from build123d import *

# Parameters (mm, degrees)
BASPROSKE_W         = 4.7625
BASPROSKE_H         = 14
TOOTHCUT_DEPTH      = 21.36372771
TEETHCUTS_COUNT     = 12
TEETHCUTS_ANGLE     = 330
BORSKE_R            = 2.6035
BORE_DEPTH          = 50.0000508
BOSS_EXTRUDE1_DEPTH = 13.99999994
SKETCH2_R           = 2.6035
CUT_EXTRUDE1_DEPTH  = 27.882327142
SKETCH3_R           = 2.5019
CUT_EXTRUDE2_DEPTH  = 32.693338104


with BuildPart() as part:
    # BasProSke → Base-Revolve (revolve)
    with BuildSketch(Plane(origin=(0, 0, 0), x_dir=(1, 0, 0), z_dir=(0, 1, 0)), mode=Mode.PRIVATE) as base_revolve_sk:
        with Locations((2.38125, 7)):
            Rectangle(BASPROSKE_W, BASPROSKE_H)
    revolve(base_revolve_sk.sketch.rotate(Axis((-10, 0, 0), (1, 0, 0)), 180), axis=Axis((-10, 0, 0), (1, 0, 0)))

    # TooCutSke → ToothCut (cut, through all)
    with BuildSketch(Plane(origin=(0, 0, 0), x_dir=(0, 0, -1), z_dir=(1, 0, 0))):
        with BuildLine():
            ThreePointArc((1.111908866, 9.433698091), (0, 9.499), (-1.111908866, 9.433698091))
            ThreePointArc((-1.111908866, 9.433698091), (-1.651516138, 11.821129337), (-3.298149691, 13.632096456))
            ThreePointArc((-3.298149691, 13.632096456), (0, 14.0254), (3.298149691, 13.632096456))
            ThreePointArc((3.298149691, 13.632096456), (1.651516138, 11.821129337), (1.111908866, 9.433698091))
        make_face()
    toothcut = extrude(amount=TOOTHCUT_DEPTH, mode=Mode.SUBTRACT)

    # TeethCuts: ToothCut ×12 about axis
    teethcuts_axis = Axis((-10, 0, 0), (1, 0, 0))
    for i in range(1, TEETHCUTS_COUNT):
        add(toothcut.rotate(teethcuts_axis, i * TEETHCUTS_ANGLE / (TEETHCUTS_COUNT - 1)), mode=Mode.SUBTRACT)

    # BorSke → Bore (cut, symmetric)
    with BuildSketch(Plane(origin=(0, 0, 0), x_dir=(0, 0, -1), z_dir=(1, 0, 0))):
        with Locations(Location((0, 0, 0), (0, 0, 180))):
            Circle(BORSKE_R)
    extrude(amount=BORE_DEPTH, both=True, mode=Mode.SUBTRACT)

    # Sketch1 → Boss-Extrude1 (add)
    with BuildSketch(Plane(origin=(4.7625, 0, 0), x_dir=(0, 0, -1), z_dir=(1, 0, 0))):
        with BuildLine():
            Line((-8, 4.618802154), (-8, -4.618802154))
            ThreePointArc((-8, -4.618802154), (0, -9.237604307), (8, -4.618802154))
            Line((8, -4.618802154), (8, 4.618802154))
            ThreePointArc((8, 4.618802154), (0, 9.237604307), (-8, 4.618802154))
        make_face()
    extrude(amount=BOSS_EXTRUDE1_DEPTH)

    # Sketch2 → Cut-Extrude1 (cut, through all)
    with BuildSketch(Plane(origin=(18.76249994, 0, 0), x_dir=(0, 0, -1), z_dir=(1, 0, 0))):
        Circle(SKETCH2_R)
    extrude(amount=-CUT_EXTRUDE1_DEPTH, mode=Mode.SUBTRACT)

    # Sketch3 → Cut-Extrude2 (cut, through all)
    with BuildSketch(Plane.XY.offset(8)):
        with Locations((11.76249997, 0)):
            Circle(SKETCH3_R)
    extrude(amount=-CUT_EXTRUDE2_DEPTH, mode=Mode.SUBTRACT)


solid = part.part
Could you check a few things on this model? Use its own coordinates, in mm. Give positions to 0.01 mm unless a question says otherwise; leave off trailing zeros. Order: outer loops, then holes, each group sorted by start corner. A loop starts at its lowest first (then second) coordinate and runs counter-clockwise, first axis right, second up. Notation, with made-up numbers: (78.25, -36) - (107.25, -36) arc R8 ccw to (107.25, -24) - close; hole circle Ø4 at (-5.5, 41.25). An arc over 180 degrees is marked (long way). Return JSON: item names as keys, results as strings. Group by question number.
Q1. Suppose I cut it at D-D, the plane x = 10. Please give me the cut outline in (y, z), and give its area (3 significant figures).
Q2. Please list where these lines run through material, in increasing order: line 1 along X through (y, z) = (0, -5.25); line 2 along Y through (x, z) = (1.25, 2); line 3 along Y through (x, z) = (1.5, -2.25). Write a range as [from, to].
Q3. Will these pins go through, and if not, where does the flat tip stop? pin 1 Ø7.5 at (x, y) = (10.5, -0.5) entering from -Z; pin 2 Ø3 at (x, y) = (15.5, 9.5) entering from +Z; pin 3 Ø4.5 at (x, y) = (11.5, 1) entering from +Z.
Q4. Suppose I cut it at C-C, the plane z = 1.5. Please give me the cut outline in (x, y) (1 decimal).
Q5. Thinking about a two-plate mould opening in Z: for faces 1 (the face through (2.348, 9.384, 7.297)), 2 (the face through (10, 2, 8)), 3 (the face through (0, -3, 0)), which applies, pulls with the +Z half, pulls with the -Z half, needs draft (parallel to the pull), parting line crosses it, or undercut?
Q6. Suppose I cut it at A-A, the plane y = 0. Please give me the cut outline in (x, z).
Q7. Suppose I cut it at B-B, the plane x = 16.75. Please give me the cut outline in (y, z), and give its area (3 significant figures).
Resolved:
{
 "1": {"outline": "(-4.62, -8) - (-1.78, -8) - (-1.78, -1.9) arc R2.6 cw to (-1.78, 1.9) - (-1.78, 8) - (-4.62, 8) arc R9.24 ccw to start; (1.78, -8) - (4.62, -8) arc R9.24 ccw to (4.62, 8) - (1.78, 8) - (1.78, 1.9) arc R2.6 cw to (1.78, -1.9) - close", "area": "191 mm2"},
 "2": {"line 1": "x = [0, 9.26], [14.26, 18.76]", "line 2": "y = [-12.39, -1.67], [1.67, 12.39]", "line 3": "y = [-12.71, -1.31], [1.31, 12.71]"},
 "3": {"pin 1": "stops at z = -8", "pin 2": "stops at z = 4.62", "pin 3": "stops at z = 8"},
 "4": {"outline": "(0, -11.5) - (4.8, -11.5) - (4.8, -9.1) - (18.8, -9.1) - (18.8, -2.1) - (13.1, -2.1) arc R2.5 cw to (10.4, -2.1) - (0, -2.1) - close; (0, 2.1) - (10.4, 2.1) arc R2.5 cw to (13.1, 2.1) - (18.8, 2.1) - (18.8, 9.1) - (4.8, 9.1) - (4.8, 11.5) - (0, 11.5) - close"},
 "5": {"face 1": "undercut", "face 2": "pulls with the +Z half", "face 3": "needs draft"},
 "6": {"outline": "(0, -9.5) - (4.76, -9.5) - (4.76, -8) - (9.26, -8) - (9.26, -2.6) - (0, -2.6) - close; (0, 2.6) - (9.26, 2.6) - (9.26, 8) - (4.76, 8) - (4.76, 9.5) - (0, 9.5) - close; (14.26, -8) - (18.76, -8) - (18.76, -2.6) - (14.26, -2.6) - close; (14.26, 2.6) - (18.76, 2.6) - (18.76, 8) - (14.26, 8) - close"},
 "7": {"outline": "(-4.62, -8) - (4.62, -8) arc R9.24 ccw to (4.62, 8) - (-4.62, 8) arc R9.24 ccw to start; hole circle Ø5.21 at (0, 0)", "area": "231 mm2"}
}
